CAD build for the part. Positions are in the model's coordinates, mm. Face numbers are marked on the shaded views. A direction names the side the tool comes from. Round coordinates to 2 decimals unless told otherwise and drop trailing zeros. Loops run counter-clockwise (first coordinate to the right, second up) from the corner with the lowest first, then second, coordinate; pieces in that order, holes last.
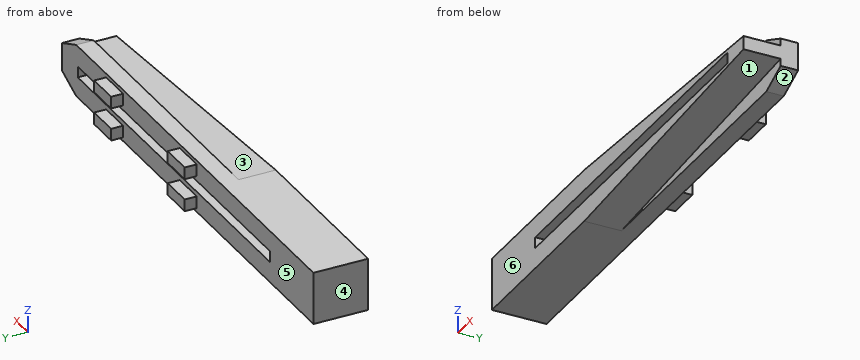
from build123d import *

# Parameters (mm, degrees)
BOSS_EXTRUDE1_DEPTH = 5
SKETCH2_W           = 169.901358226
SKETCH2_H           = 5.057880692
CUT_EXTRUDE1_DEPTH  = 26
SKETCH3_W           = 15
SKETCH3_H           = 5.5
BOSS_EXTRUDE2_DEPTH = 5.5
SKETCH4_W           = 169.901358226
SKETCH4_H           = 5.057880692
BOSS_EXTRUDE3_DEPTH = 20
CUT_EXTRUDE5_DEPTH  = 17


with BuildPart() as part:
    # Sketch1 → Boss-Extrude1 (new body)
    with BuildSketch(Plane(origin=(0, 0, 0), x_dir=(1, 0, 0), z_dir=(0, 1, 0))):
        Polygon((-69.180780697, 17.519952768), (140.433207055, 17.519952768), (153.094163244, 11.942432967), (153.094163244, -0.867190791), (140.433207055, -6.444710592), (-69.180780697, -6.444710592), align=None)
    extrude(amount=BOSS_EXTRUDE1_DEPTH)

    # Sketch2 → Cut-Extrude1 (cut)
    with BuildSketch(Plane.XZ):
        with Locations((54.091074894, -5.537621088)):
            Rectangle(SKETCH2_W, SKETCH2_H)
    extrude(amount=-CUT_EXTRUDE1_DEPTH, mode=Mode.SUBTRACT)

    # Sketch3 → Boss-Extrude2 (add)
    with BuildSketch(Plane(origin=(0, 5, 0), x_dir=(1, 0, 0), z_dir=(0, 1, 0))):
        with Locations((106.456138521, 13.037621088)):
            Rectangle(SKETCH3_W, SKETCH3_H)
        with Locations((106.456138521, -1.962378912)):
            Rectangle(SKETCH3_W, SKETCH3_H)
        with Locations((41.456138521, -1.962378912)):
            Rectangle(SKETCH3_W, SKETCH3_H)
        with Locations((41.456138521, 13.037621088)):
            Rectangle(SKETCH3_W, SKETCH3_H)
    extrude(amount=BOSS_EXTRUDE2_DEPTH)

    # Sketch4 → Boss-Extrude3 (add)
    with BuildSketch(Plane.XZ):
        Polygon((-69.180780697, 6.444710592), (-69.180780697, -17.519952768), (140.433207055, -17.519952768), (153.094163244, -11.942432967), (153.094163244, 0.867190791), (140.433207055, 6.444710592), align=None)
        with Locations((54.091074894, -5.537621088)):
            Rectangle(SKETCH4_W, SKETCH4_H, mode=Mode.SUBTRACT)
    extrude(amount=BOSS_EXTRUDE3_DEPTH)

    # Sketch7 → Cut-Extrude5 (cut)
    with BuildSketch(Plane.XZ.offset(20)):
        Polygon((12.387057353, -17.519952768), (140.433207055, -17.519952768), (153.094163244, -11.942432967), (153.094163244, -8.637621088), align=None)
        Polygon((153.094163244, -2.437621088), (153.094163244, 0.867190791), (140.433207055, 6.444710592), (12.387057353, 6.444710592), align=None)
    extrude(amount=-CUT_EXTRUDE5_DEPTH, mode=Mode.SUBTRACT)


solid = part.part
Item 1: Flat gauge pins, fed straight in: P1, Ø1.6, axis at y = 7.5, z = -14, coming from the +X side; P2, Ø1.5, axis at x = 25, z = -10, coming from the +Y side; P3, Ø4, axis at x = 52, y = -7.5, coming from the -Z side; P4, Ø4, axis at x = -46, y = 7.5, coming from the -Z side. Where does each tip first touch, or does it go through?
Verdict:
P1: stops at x = 113.96
P2: stops at y = 5
P3: stops at z = -15.15
P4: passes through
Item 2: Mould opens along X. For the marked faces 4, 5 and 6 say: released by +X, released by -X, zero draft, split by the parting line, or undercut.
Verdict:
face 4: released by -X
face 5: undercut
face 6: zero draft
Item 3: Cut at D-D (x = 21). List the corners of the cut face in (y, z), plus the area to 3 significant figures.
Verdict:
outline: (-20, -16.98) - (-3, -16.98) - (-3, -17.52) - (5, -17.52) - (5, -8.07) - (-20, -8.07) - close; (-20, -3.01) - (5, -3.01) - (5, 6.44) - (-3, 6.44) - (-3, 5.9) - (-20, 5.9) - close
area: 454 mm2
Item 4: Cut at C-C (y = -17.5). List the corners of the cut face in (x, z), plus the area to 3 significant figures.
Verdict:
outline: (-69.18, -17.52) - (12.39, -17.52) - (153.09, -8.64) - (153.09, -2.44) - (12.39, 6.44) - (-69.18, 6.44) - close; hole (-30.86, -8.07) - (139.04, -8.07) - (139.04, -3.01) - (-30.86, -3.01) - close
area: 3,220 mm2
Item 5: 3-axis set-ups, long thin cutter, end or side, ignore diameter. For the marked faces 1, 2 and 3: which of +Z, -Z, +X, -X, +Y, -Y reach the whole face in a straight line?
Verdict:
face 1: -Z, +X, -Y
face 2: -Z, +X, +Y, -Y
face 3: +Z, +X, -Y
Item 6: Wall check: L1, parallel to Z at x = 39, y = -2; L2, parallel to X at y = -12.5, z = -6.5; L3, parallel to Y at x = 139, z = -11.75. Give the ranges that are in metal, low to high.
Verdict:
L1: z = -17.52 to -8.07, -3.01 to 6.44
L2: x = -69.18 to -30.86, 139.04 to 153.09
L3: y = -3 to 5
Item 7: Cut at B-B (y = 7.5). List the corners of the cut face in (x, z).
Verdict:
outline: (33.96, -15.79) - (48.96, -15.79) - (48.96, -10.29) - (33.96, -10.29) - close; (33.96, -0.79) - (48.96, -0.79) - (48.96, 4.71) - (33.96, 4.71) - close; (98.96, -15.79) - (113.96, -15.79) - (113.96, -10.29) - (98.96, -10.29) - close; (98.96, -0.79) - (113.96, -0.79) - (113.96, 4.71) - (98.96, 4.71) - close
Item 8: Cut at A-A (x = -28.5). List the corners of the cut face in (y, z), plus the area to 3 significant figures.
Verdict:
outline: (-20, -17.52) - (5, -17.52) - (5, -8.07) - (-20, -8.07) - close; (-20, -3.01) - (5, -3.01) - (5, 6.44) - (-20, 6.44) - close
area: 473 mm2
